Here's the drawing with two shaded views (mm, measured from the low corner). I have some questions. Give positions to 0.01 mm unless a question says otherwise; leave off trailing zeros. Order: outer loops, then holes, each group sorted by start corner. A loop starts at its lowest first (then second) coordinate and runs counter-clockwise, first axis right, second up. Notation, with made-up numbers: M -18.75,42.5 L 7.25,42.5 A33 ccw 7.25,70.5 Z; hole C 50,-21.5 d1. An arc over 180 degrees is marked long. Use a Markdown table: item, result. Add a question column.
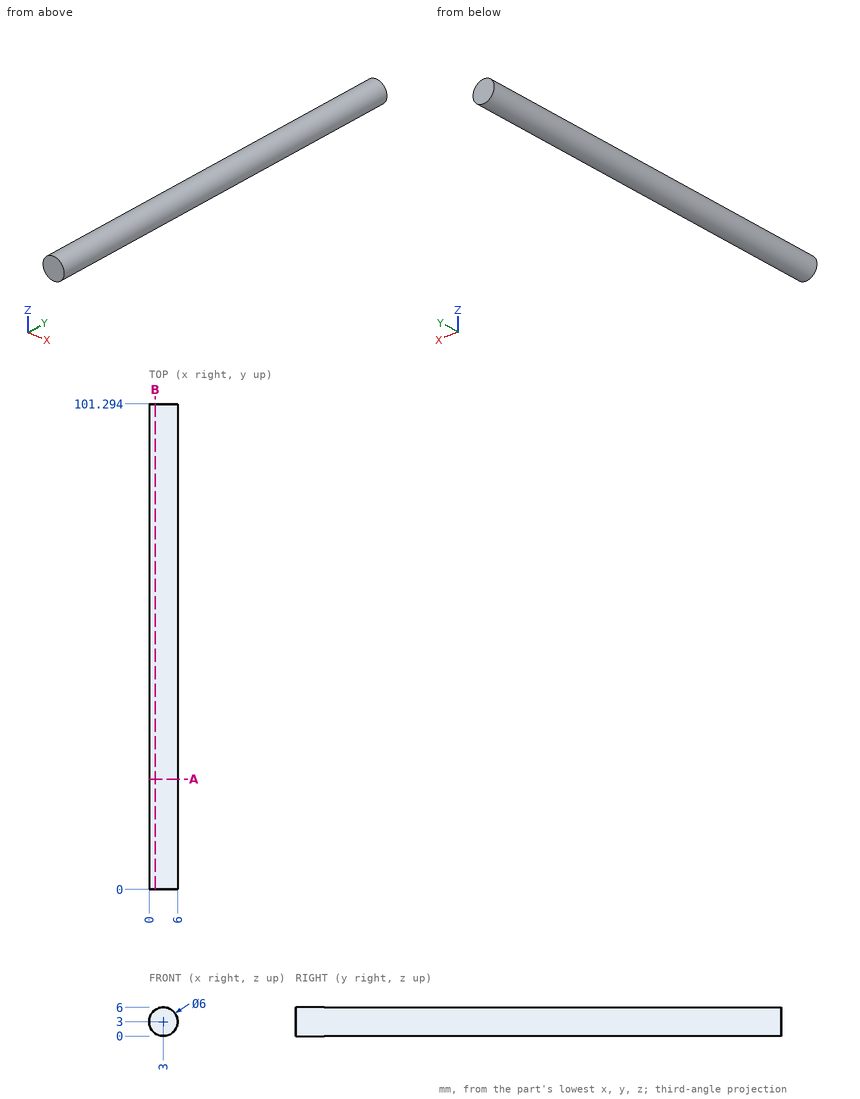
1) Suppose I cut it at B-B on x = 1.3. Please give me the cut outline in (y, z), and give its area (3 significant figures).
2) For pin 1 (3 mm diameter, centred on x = 1, y = 85.5, fed in from -Z); pin 2 (2 mm diameter, centred on x = 1.5, y = 16.5, fed in from +Z); pin 3 (1 mm diameter, centred on x = 1, y = 16.5, fed in from -Z), each with a flat end and sliding along its axis, tell me the tip position at first contact or that it passes through.
3) Suppose I cut it at A-A on y = 23. Please give me the cut outline in (x, z), and give its area (3 significant figures).
4) Please list where these lines run through material, in increasing order: line 1 (Z direction, x = 2.85, y = 13); line 2 (Z direction, x = 1.3, y = 13). Write a range as from..to.
Values found:
| question | item | result |
|---|---|---|
| 1 | outline | M 0,0.53 L 101.29,0.53 L 101.29,5.47 L 0,5.47 Z |
| 1 | area | 501 mm^2 |
| 2 | pin 1 | stops at z = 0.04 |
| 2 | pin 2 | stops at z = 5.96 |
| 2 | pin 3 | stops at z = 0.4 |
| 3 | outline | C 3,3 d6 |
| 3 | area | 28.3 mm^2 |
| 4 | line 1 | z = 0..6 |
| 4 | line 2 | z = 0.53..5.47 |
